from build123d import *

# Parameters (mm, degrees)
SKETCH2_W           = 5
SKETCH2_H           = 3
BOSS_EXTRUDE1_DEPTH = 15
SKETCH3_R           = 15
SKETCH3_R_2         = 3.5
BOSS_EXTRUDE2_DEPTH = 3
BOSS_EXTRUDE3_START = 3
SKETCH4_R           = 15
SKETCH4_R_2         = 3.5
BOSS_EXTRUDE3_DEPTH = 3


# Read off the part's stored shape, not the designer's step: Pulley part01 GT2 6mm.STEP
with BuildPart() as part:
    # Sketch2 → Boss-Extrude1 (new body)
    with BuildSketch(Plane.XY.offset(5)):
        with BuildLine():
            ThreePointArc((6.934106351, 5.59049504), (7.051433078, 7.907185894), (4.763236954, 7.526422749))
            ThreePointArc((4.763236954, 7.526422749), (3.583838208, 8.154236284), (2.32379934, 8.598570946))
            ThreePointArc((2.32379934, 8.598570946), (1.057001937, 10.541776134), (-0.570380652, 8.888764346))
            ThreePointArc((-0.570380652, 8.888764346), (-1.893553819, 8.703442975), (-3.174120037, 8.322285003))
            ThreePointArc((-3.174120037, 8.322285003), (-5.341168017, 9.149766191), (-5.686132237, 6.855900077))
            ThreePointArc((-5.686132237, 6.855900077), (-6.647672646, 5.928230265), (-7.459633444, 4.86716905))
            ThreePointArc((-7.459633444, 4.86716905), (-9.699193326, 4.262856549), (-8.629974569, 2.204315))
            ThreePointArc((-8.629974569, 2.204315), (-8.862606466, 0.888635084), (-8.895820416, -0.447040053))
            ThreePointArc((-8.895820416, -0.447040053), (-10.352456447, -2.252319406), (-8.277459935, -3.289243485))
            ThreePointArc((-8.277459935, -3.289243485), (-7.692325842, -4.490388494), (-6.934106344, -5.590495048))
            ThreePointArc((-6.934106344, -5.590495048), (-7.05143307, -7.907185904), (-4.763236946, -7.526422754))
            ThreePointArc((-4.763236946, -7.526422754), (-3.583838199, -8.154236288), (-2.323799332, -8.598570948))
            ThreePointArc((-2.323799332, -8.598570948), (-1.057001929, -10.541776143), (0.570380658, -8.888764345))
            ThreePointArc((0.570380658, -8.888764345), (1.893553823, -8.703442974), (3.174120041, -8.322285002))
            ThreePointArc((3.174120041, -8.322285002), (5.341168023, -9.149766199), (5.686132236, -6.855900078))
            ThreePointArc((5.686132236, -6.855900078), (6.647672645, -5.928230266), (7.459633443, -4.867169052))
            ThreePointArc((7.459633443, -4.867169052), (9.699193332, -4.262856559), (8.629974567, -2.204315006))
            ThreePointArc((8.629974567, -2.204315006), (8.862606465, -0.888635092), (8.895820416, 0.447040044))
            ThreePointArc((8.895820416, 0.447040044), (10.352456454, 2.252319396), (8.277459939, 3.289243476))
            ThreePointArc((8.277459939, 3.289243476), (7.692325847, 4.490388485), (6.934106351, 5.59049504))
        make_face()
        Rectangle(SKETCH2_W, SKETCH2_H, mode=Mode.SUBTRACT)
    extrude(amount=BOSS_EXTRUDE1_DEPTH)

    # Sketch3 → Boss-Extrude2 (add)
    with BuildSketch(Plane(origin=(0, 0, 5), x_dir=(-1, 0, 0), z_dir=(0, 0, -1))):
        Circle(SKETCH3_R)
        Circle(SKETCH3_R_2, mode=Mode.SUBTRACT)
    extrude(amount=BOSS_EXTRUDE2_DEPTH)

    # Sketch4 → Boss-Extrude3 (add)
    with BuildSketch(Plane.XY.offset(20).offset(BOSS_EXTRUDE3_START)):
        with Locations(Location((0, 0, 0), (0, 0, 180))):
            Circle(SKETCH4_R)
        with Locations(Location((0, 0, 0), (0, 0, 180))):
            Circle(SKETCH4_R_2, mode=Mode.SUBTRACT)
    extrude(amount=-BOSS_EXTRUDE3_DEPTH)


solid = part.part
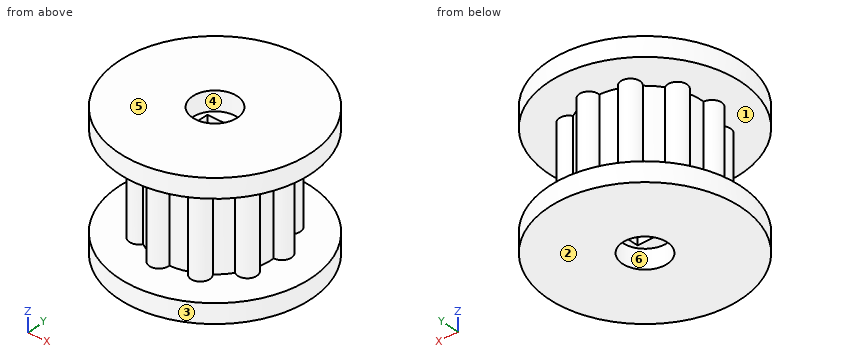
Could you check a few things on this model? Use its own coordinates, in mm. Face numbers are marked on the shaded views. A direction names the side the tool comes from. Round coordinates to 2 decimals unless told otherwise and drop trailing zeros. Order: outer loops, then holes, each group sorted by start corner. A loop starts at its lowest first (then second) coordinate and runs counter-clockwise, first axis right, second up. Notation, with made-up numbers: M -34.75,43 L -18.75,43 A25 cw -18.75,69 Z; hole C -19,23.25 d2. An arc over 180 degrees is marked long. One line per item, written item: value.
(1) Which directions (+Z, -Z, +X, -X, +Y, -Y) give clear straight access to the entire face, cutting with the end or side of a thin tool? Please do the marked faces 1 and 2.
Ans:
face 1: none
face 2: -Z, +X, -X, +Y, -Y
(2) Imagine slicing it at A-A (y = 0). Write out the boundary of the cut face in (x, z).
Ans:
outline: M -15,2 L -3.5,2 L -3.5,5 L -2.5,5 L -2.5,20 L -3.5,20 L -3.5,23 L -15,23 L -15,20 L -8.91,20 L -8.91,5 L -15,5 Z; M 2.5,5 L 3.5,5 L 3.5,2 L 15,2 L 15,5 L 8.91,5 L 8.91,20 L 15,20 L 15,23 L 3.5,23 L 3.5,20 L 2.5,20 Z
(3) I need wall thicknesses on line 1 along Y through (x, z) = (0, 4.3); line 2 along Z through (x, y) = (9, -5.5); line 3 along X through (y, z) = (0, 13.25). Which ranges of each line are inside material? Lowest first, please. Write a range as from..to.
Ans:
line 1: y = -15..-3.5, 3.5..15
line 2: z = 2..5, 20..23
line 3: x = -8.91..-2.5, 2.5..8.91
(4) If we mould it in two halves opening along Y, with no side actions, what happens to the marked faces 3, 4, 5 and 6? For each: released by +Y, released by -Y, zero draft, split by the parting line, or undercut.
Ans:
face 3: split by the parting line
face 4: undercut
face 5: zero draft
face 6: undercut
(5) Imagine slicing it at C-C (z = 7.5). Write out the boundary of the cut face in (x, y), and give its area (3 significant figures).
Ans:
outline: M -8.9,-0.45 A1.49 ccw long -8.28,-3.29 A8.91 ccw -6.93,-5.59 A1.49 ccw long -4.76,-7.53 A8.91 ccw -2.32,-8.6 A1.49 ccw long 0.57,-8.89 A8.91 ccw 3.17,-8.32 A1.49 ccw long 5.69,-6.86 A8.91 ccw 7.46,-4.87 A1.49 ccw long 8.63,-2.2 A8.91 ccw 8.9,0.45 A1.49 ccw long 8.28,3.29 A8.91 ccw 6.93,5.59 A1.49 ccw long 4.76,7.53 A8.91 ccw 2.32,8.6 A1.49 ccw long -0.57,8.89 A8.91 ccw -3.17,8.32 A1.49 ccw long -5.69,6.86 A8.91 ccw -7.46,4.87 A1.49 ccw long -8.63,2.2 A8.91 ccw Z; hole M -2.5,-1.5 L 2.5,-1.5 L 2.5,1.5 L -2.5,1.5 Z
area: 276 mm^2
(6) I'm going to push flat-ended pins straight in: P1, Ø1.5, axis at y = 0, z = 16, coming from the -X side; P2, Ø8, axis at y = -8, z = 5, coming from the +X side; P3, Ø2.5, axis at x = -0.5, z = 9, coming from the +Y side. Where does each tip first touch, or does it pass through?
Ans:
P1: stops at x = -9.8
P2: stops at x = 14.46
P3: stops at y = 10.54
(7) Imagine slicing it at B-B (x = 0). Write out the boundary of the cut face in (y, z).
Ans:
outline: M -15,2 L -3.5,2 L -3.5,5 L -1.5,5 L -1.5,20 L -3.5,20 L -3.5,23 L -15,23 L -15,20 L -10.24,20 L -10.24,5 L -15,5 Z; M 1.5,5 L 3.5,5 L 3.5,2 L 15,2 L 15,5 L 10.24,5 L 10.24,20 L 15,20 L 15,23 L 3.5,23 L 3.5,20 L 1.5,20 Z
(8) Imagine slicing it at D-D (x = -5.25). Write out the boundary of the cut face in (y, z).
Ans:
outline: M -14.05,2 L 14.05,2 L 14.05,5 L 9.2,5 L 9.2,20 L 14.05,20 L 14.05,23 L -14.05,23 L -14.05,20 L -8.04,20 L -8.04,5 L -14.05,5 Z
